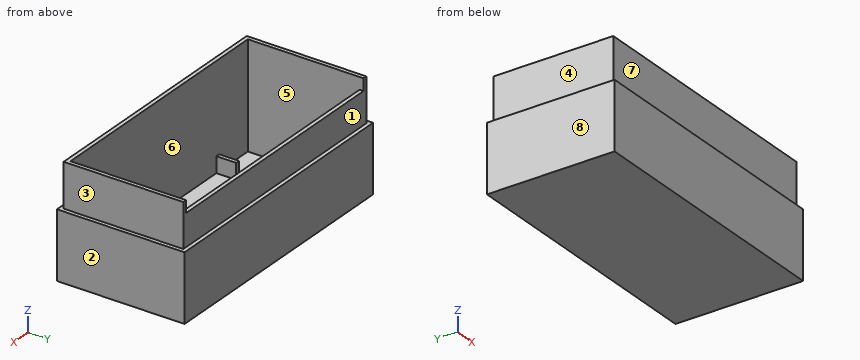
```python
from build123d import *

# Parameters (mm, degrees)
F0_W     = 67.5
F0_H     = 32
F1_DEPTH = 1.5
F2_W     = 67.5
F2_H     = 32
F2_W_2   = 63.5
F2_H_2   = 28
F3_DEPTH = 26.3
F4_W     = 63.5
F4_H     = 2
F5_DEPTH = 3
F6_W     = 67.5
F6_H     = 32
F6_W_2   = 65.5
F6_H_2   = 30
F7_DEPTH = 11
F8_W     = 5
F8_H     = 1
F8_W_2   = 1
F8_H_2   = 5
F9_DEPTH = 4


with BuildPart() as f1:
    # F0 (on Top) → F1 (new body)
    with BuildSketch(Plane.XY):
        with Locations((33.75, 16)):
            Rectangle(F0_W, F0_H)
    extrude(amount=F1_DEPTH)

    # F2 (on face) → F3 (join)
    with BuildSketch(Plane.XY.offset(1.5)):
        with Locations((33.75, 16)):
            Rectangle(F2_W, F2_H)
        with Locations((33.75, 16)):
            Rectangle(F2_W_2, F2_H_2, mode=Mode.SUBTRACT)
    extrude(amount=F3_DEPTH)

    # F4 (on face) → F5 (cut)
    with BuildSketch(Plane.XY.offset(27.8)):
        with Locations((33.75, 31)):
            Rectangle(F4_W, F4_H)
    extrude(amount=-F5_DEPTH, mode=Mode.SUBTRACT)

    # F6 (on face) → F7 (cut)
    with BuildSketch(Plane.XY.offset(27.8)):
        with Locations((33.75, 16)):
            Rectangle(F6_W, F6_H)
        with Locations((33.75, 16)):
            Rectangle(F6_W_2, F6_H_2, mode=Mode.SUBTRACT)
    extrude(amount=-F7_DEPTH, mode=Mode.SUBTRACT)

    # F8 (on face) → F9 (join)
    with BuildSketch(Plane.XY.offset(1.5)):
        with Locations((63, 13.8)):
            Rectangle(F8_W, F8_H)
        with Locations((12.8, 27.5)):
            Rectangle(F8_W_2, F8_H_2)
        with Locations((12.8, 4.5)):
            Rectangle(F8_W_2, F8_H_2)
    extrude(amount=F9_DEPTH)


solid = f1.part
```
For this review, take the finished solid that the model builds, in its own axes (mm). Face numbers are marked on the shaded views. A direction names the side the tool comes from. Coordinates: 2 decimals unless noted, no trailing zeros. Loops run counter-clockwise (first coordinate to the right, second up) from the corner with the lowest first, then second, coordinate; pieces in that order, holes last.
1. Add section B-B, the plane y = 18. Give the boundary of the cut face in (x, z), then the cut area to 3 significant figures.
2. For the marked faces 1, 2, 3, 4 and 5, list the 3-axis set-ups (+Z, -Z, +X, -X, +Y, -Y) from which the entire face can be reached by the end or side of a thin tool; tool diameter is ignored.
3. Add section C-C, the plane z = 25.75. Give the boundary of the cut face in (x, y), then the cut area to 4 significant figures.
4. Insertion check: P1, Ø8.5, axis at x = 28, y = 18, coming from the +Z side; P2, Ø5, axis at x = 56.5, z = 23.5, coming from the -Y side; P3, Ø10, axis at x = 9, y = 22.5, coming from the +Z side. Each pin has a flat end and moves straight along its axis. Give the tip position at first contact, or say it passes through.
5. Add section D-D, the plane x = 51.5. Give the boundary of the cut face in (y, z), then the cut area to 3 significant figures.
6. Mouldability with a two-part tool opening along X and no side actions: class the marked faces 6, 7 and 8 as +X half, -X half, draft (parallel to the pull), parting line (faces both ways), or undercut.
7. For line 1 (Y direction, x = 57, z = 21); line 2 (Y direction, x = 63, z = 4.25); line 3 (Y direction, x = 45.5, z = 4), list the stretches that pass through material, from the lowest coordinate up.
8. Add section A-A, the plane z = 20. Give the boundary of the cut face in (x, y).
Result:
1. outline: (0, 0) - (67.5, 0) - (67.5, 16.8) - (66.5, 16.8) - (66.5, 27.8) - (65.5, 27.8) - (65.5, 1.5) - (2, 1.5) - (2, 27.8) - (1, 27.8) - (1, 16.8) - (0, 16.8) - close
1. area: 184 mm2
2. face 1: +Z, +X, -X, +Y
2. face 2: +Z, -Z, +X, +Y, -Y
2. face 3: +Z, +X, +Y, -Y
2. face 4: +Z, -X, +Y, -Y
2. face 5: +Z
3. outline: (1, 1) - (66.5, 1) - (66.5, 31) - (65.5, 31) - (65.5, 2) - (2, 2) - (2, 31) - (1, 31) - close
3. area: 123.5 mm2
4. P1: stops at z = 1.5
4. P2: stops at y = 1
4. P3: stops at z = 5.5
5. outline: (0, 0) - (32, 0) - (32, 16.8) - (31, 16.8) - (31, 24.8) - (30, 24.8) - (30, 1.5) - (2, 1.5) - (2, 27.8) - (1, 27.8) - (1, 16.8) - (0, 16.8) - close
5. area: 128 mm2
6. face 6: undercut
6. face 7: draft
6. face 8: -X half
7. line 1: y = 1 to 2, 30 to 31
7. line 2: y = 0 to 2, 13.3 to 14.3, 30 to 32
7. line 3: y = 0 to 2, 30 to 32
8. outline: (1, 1) - (66.5, 1) - (66.5, 31) - (1, 31) - close; hole (2, 2) - (65.5, 2) - (65.5, 30) - (2, 30) - close
